from build123d import *


with BuildPart() as part:
    # Sketch1 → Revolve1 (revolve)
    with BuildSketch(Plane.XY, mode=Mode.PRIVATE) as revolve1_sk:
        with BuildLine():
            Line((3.4925, -11.813333327), (3.4925, 28.88))
            ThreePointArc((3.4925, 28.88), (3.937697693, 29.954802307), (5.0125, 30.4))
            Line((5.0125, 30.4), (27.08, 30.4))
            ThreePointArc((27.08, 30.4), (28.154802307, 29.954802307), (28.6, 28.88))
            Line((28.6, 28.88), (28.6, 0))
            Line((28.6, 0), (27.172081158, 0))
            ThreePointArc((27.172081158, 0), (26.767558692, -0.167558692), (26.6, -0.572081158))
            Line((26.6, -0.572081158), (26.6, -11.813333327))
            ThreePointArc((26.6, -11.813333327), (26.154802307, -12.888135634), (25.08, -13.333333327))
            Line((25.08, -13.333333327), (5.0125, -13.333333327))
            ThreePointArc((5.0125, -13.333333327), (3.937697693, -12.888135634), (3.4925, -11.813333327))
        make_face()
    revolve(revolve1_sk.sketch.rotate(Axis((0, 0, 0), (0, 1, 0)), 90), axis=Axis((0, 0, 0), (0, 1, 0)))


solid = part.part
The listing builds one solid part. Answer for the finished solid, in the listing's coordinates (mm). A direction names the side the tool comes from. Round coordinates to 2 decimals unless told otherwise and drop trailing zeros. Write each loop counter-clockwise with the first axis right and the second up, starting at its lowest first coordinate (ties: lowest second). Pieces come first, ordered by that corner, then holes. Notation, with made-up numbers: M 61.25,-30.5 L 70.25,-30.5 A19 ccw 70.25,-12.5 Z; hole C -7.5,1.5 d6. An arc over 180 degrees is marked long. Write each question's results on one line, items separated by ' | '. Start each with the question number.
(1) The part is cut by section D-D, the plane y = -6. Write down the section's boundary in (x, z) (1 decimal), and give its area (3 significant figures).
(2) Each of these flat-tipped pins is pushed along its axis until it touches: P1, Ø5, axis at y = 8.5, z = -18, coming from the +X side; P2, Ø4, axis at y = 23, z = 22, coming from the +X side; P3, Ø2, axis at x = -22, y = 11, coming from the +Z side; P4, Ø6.5, axis at x = 0, z = 0, coming from the +Y side. Where does it stop, or does it pass through?
(3) Find the intervals of material crossed by line 1 (X direction, y = 12, z = 0); line 2 (X direction, y = -3, z = 0); line 3 (Y direction, x = -19.5, z = -16), in increasing order.
(4) The part is cut by section A-A, the plane z = 0. Write down the section's boundary in (x, y).
(5) For faces 1 (the cylindrical face through (-28.357, 14.238, 3.723)), 2 (the flat face through (10.5, 0, -25.3)), determine the directions among +Z, -Z, +X, -X, +Y, -Y from which every point of the face is accessible in a straight line to the end or side of a thin tool.
(6) The part is cut by section C-C, the plane y = 21. Write down the section's boundary in (x, z) (1 decimal), and give its area (3 significant figures).
(7) The part is cut by section B-B, the plane x = 0. Write down the section's boundary in (y, z).
(8) Determine the mould class of faces 3 (the flat face through (6, 30.4, 0)), 4 (the cylindrical face through (25.967, -6.271, 5.766)), 5 (the cylindrical face through (-3.463, 8.818, 0.455)) for opening direction X: +X half, -X half, draft (parallel to the pull), parting line (faces both ways), or undercut.
Worked answers:
1) outline: C 0,0 d53.2; hole C 0,0 d7 | area: 2,180 mm²
2) P1: stops at x = 24.04 | P2: stops at x = 20.44 | P3: stops at z = 19.42 | P4: passes through
3) line 1: x = -28.6 to -3.49, 3.49 to 28.6 | line 2: x = -26.6 to -3.49, 3.49 to 26.6 | line 3: y = -13.33 to 30.4
4) outline: M -28.6,0 L -27.17,0 A0.57 cw -26.6,-0.57 L -26.6,-11.81 A1.52 ccw -25.08,-13.33 L -5.01,-13.33 A1.52 ccw -3.49,-11.81 L -3.49,28.88 A1.52 ccw -5.01,30.4 L -27.08,30.4 A1.52 ccw -28.6,28.88 Z; M 3.49,-11.81 A1.52 ccw 5.01,-13.33 L 25.08,-13.33 A1.52 ccw 26.6,-11.81 L 26.6,-0.57 A0.57 cw 27.17,0 L 28.6,0 L 28.6,28.88 A1.52 ccw 27.08,30.4 L 5.01,30.4 A1.52 ccw 3.49,28.88 Z
5) face 1: +Y, -Y | face 2: -Y
6) outline: C 0,0 d57.2; hole C 0,0 d7 | area: 2,530 mm²
7) outline: M -13.33,-25.08 A1.52 ccw -11.81,-26.6 L -0.57,-26.6 A0.57 cw 0,-27.17 L 0,-28.6 L 28.88,-28.6 A1.52 ccw 30.4,-27.08 L 30.4,-5.01 A1.52 ccw 28.88,-3.49 L -11.81,-3.49 A1.52 ccw -13.33,-5.01 Z; M -13.33,5.01 A1.52 ccw -11.81,3.49 L 28.88,3.49 A1.52 ccw 30.4,5.01 L 30.4,27.08 A1.52 ccw 28.88,28.6 L 0,28.6 L 0,27.17 A0.57 cw -0.57,26.6 L -11.81,26.6 A1.52 ccw -13.33,25.08 Z
8) face 3: draft | face 4: parting line | face 5: undercut
